Read the model definition and answer for the solid it produces. Units are mm, in the model's axes. Coordinates: 2 decimals unless noted, no trailing zeros. Write each loop counter-clockwise with the first axis right and the second up, starting at its lowest first coordinate (ties: lowest second). Pieces come first, ordered by that corner, then holes.
1) The part is cut by section C-C (x = -34.5). Determine the outline of the cut face in (y, z), then the cut area to 3 significant figures.
2) The part is cut by section D-D (z = 9.5). Determine the outline of the cut face in (x, y).
3) Determine the mould class of faces 1 (the face through (-42.5, 50, 16)), 2 (the face through (0.623, 50.286, 11.386)), 3 (the face through (25, 50, 32)) for opening direction X: +X half, -X half, draft (parallel to the pull), parting line (faces both ways), or undercut.
4) Find the intervals of material crossed by line 1 (X direction, y = 53, z = 26.5); line 2 (X direction, y = 10.5, z = 27); line 3 (Z direction, x = -15, y = 40), in increasing order.
5) The part is cut by section B-B (y = 85). Determine the outline of the cut face in (x, z).
6) Each of these flat-tipped pins is pushed along its axis until it touches: pin 1 Ø6 at (x, y) = (33.5, 36.5) entering from -Z; pin 2 Ø1 at (x, y) = (3.5, 10.5) entering from +Z; pin 3 Ø8 at (x, z) = (0, 11) entering from +Y. Where does it stop, or does it pass through?
Autodesk Fusion 360 part; units mm, degrees
sketch "Sketch1" plane through (0, 0, 0) normal (0, 1, 0) x (1, 0, 0)
  line L0 (-42.5, 0) -> (42.5, 0)
  line L1 (42.5, 0) -> (42.5, -32)
  line L2 (42.5, -32) -> (-42.5, -32)
  line L3 (-42.5, -32) -> (-42.5, 0)
  arc A0 (-42.5, 0) -> (42.5, 0) centre (0, 73.6122) ccw
  line L4 (-30, -32) -> (30, -32)
  line L5 (18, -20) -> (-18, -20)
  arc A1 (-18, -20) -> (-30, -32) centre (-18, -32) ccw
  arc A2 (30, -32) -> (18, -20) centre (18, -32) ccw
  arc A3 (6, -32) -> (-6, -32) centre (0, -32) ccw
  dimension "d1" = 42.5
  dimension "d2" = 42.5
  dimension "d3" = 32
  dimension "d4" = 32
  dimension "d5" = 170
  dimension "d6" = 20
  dimension "d9" = 12
  dimension "d10" = 12
  dimension "d11" = 30
  dimension "d12" = 30
  dimension "d13" = 12
  dimension "d14" = 42.5
extrude "Extrude1" add sketch "Sketch1" along normal blind 102 contours L1 L2 L3 A0 L5 A1 A2 | L2 L4 L5 A1 A2 A3
extrude "Extrude2" add sketch "Sketch1" along normal blind 73 contours L2 L4 A3
loft "Loft1" cut profiles "Sketch1" section 1 contours L2 L4 L5 A1 A2 A3 | L2 L4 A3 section 2 face at (-0.1495, 73, 30.0056)
equation "d1 = ( 85 / 2 ) * 1 mm"
equation "d2 = ( 85 / 2 ) * 1 mm"
equation "d5 = ( 85 * 2 ) * 1 mm"
equation "d14 = d2"
equation "d17 = 102 mm - 29 mm"
Reported:
1. outline: (0, 4.07) - (102, 4.07) - (102, 32) - (0, 32) - close
1. area: 2,850 mm2
2. outline: (-42.5, 0) - (-17.81, 0) - (-17.81, 102) - (-42.5, 102) - close; (17.81, 0) - (42.5, 0) - (42.5, 102) - (17.81, 102) - close
3. face 1: -X half
3. face 2: undercut
3. face 3: draft
4. line 1: x = -42.5 to -9.77, 9.77 to 42.5
4. line 2: x = -42.5 to -25.36, 25.36 to 42.5
4. line 3: z = 10.05 to 26.78, 31.47 to 32
5. outline: (-42.5, 0) arc R85 cw to (42.5, 0) - (42.5, 32) - (6, 32) arc R6 cw to (-6, 32) - (-42.5, 32) - close
6. pin 1: stops at z = 3.15
6. pin 2: stops at z = 20.92
6. pin 3: stops at y = 102
